```python
from build123d import *

# Parameters (mm, degrees)
F0_W     = 25.4
F0_H     = 25.4
F1_DEPTH = 25.4
F3_DEPTH = 25.4
F4_W     = 25.4
F4_H     = 12.7
F5_DEPTH = 25.4
F6_W     = 12.7
F6_H     = 12.7
F7_DEPTH = 25.4


with BuildPart() as f1:
    # F0 (on Front) → F1 (new body)
    with BuildSketch(Plane.XZ):
        with Locations((12.7, 12.7)):
            Rectangle(F0_W, F0_H)
    extrude(amount=F1_DEPTH)

    # F2 (on face) → F3 (cut)
    with BuildSketch(Plane.XZ.offset(25.4)):
        Polygon((5.187699, 9.677647), (0.70863, 9.677647), (0.70863, 7.712204), (1.221623, 7.712204), (1.221623, 4.225912), (0.734957, 4.225912), (0.734957, 2.289937), (3.984629, 2.289937), (3.984629, 4.225912), (3.45915, 4.225912), (3.45915, 4.571622), (5.187699, 4.571622), (6.487568, 5.940633), (6.487568, 8.277631), align=None)
        Polygon((1.373146, 8.298191), (1.373146, 9.056263), (4.895022, 9.024677), (5.842611, 8.09288), (5.842611, 6.181907), (4.942401, 5.234317), (2.826117, 5.234317), (2.826117, 3.623415), (3.284119, 3.623415), (3.284119, 2.928515), (1.373146, 2.928515), (1.373146, 3.623415), (1.89432, 3.623415), (1.89432, 8.298191), align=None, mode=Mode.SUBTRACT)
        Polygon((10.355519, 9.670121), (7.154135, 9.670121), (7.164647, 7.688757), (7.654916, 7.688757), (7.654916, 4.259461), (7.164647, 4.259461), (7.164647, 2.317117), (10.355519, 2.317117), (10.355519, 4.259461), (9.8595, 4.259461), (9.8595, 7.691912), (10.355519, 7.691912), align=None)
        Polygon((7.806116, 8.34365), (7.802438, 9.036948), (9.705184, 9.037424), (9.708923, 8.332776), (9.163893, 8.329884), (9.18893, 3.610964), (9.708865, 3.624296), (9.722495, 2.901242), (7.792784, 2.891004), (7.788839, 3.634657), (8.348879, 3.637628), (8.348879, 8.34653), align=None, mode=Mode.SUBTRACT)
        Polygon((13.681499, 9.670121), (11.003493, 9.670121), (11.003493, 7.688757), (11.510781, 7.688757), (11.510781, 4.259461), (11.003493, 4.259461), (11.003493, 2.317117), (13.988231, 2.317117), (13.988231, 4.166804), (13.351173, 4.166804), (13.351173, 5.936412), (15.344931, 2.317117), (17.279701, 2.317117), (17.279701, 7.688757), (17.810585, 7.688757), (17.810585, 9.670121), (14.908427, 9.670121), (14.908427, 7.800398), (15.403918, 7.800398), (15.403918, 6.420104), align=None)
        Polygon((11.66257, 8.332776), (11.658834, 9.036948), (13.255958, 9.006472), (15.985473, 4.235322), (15.985473, 8.338282), (15.528347, 8.332776), (15.520232, 9.006472), (17.214789, 9.026884), (17.218454, 8.336145), (16.583439, 8.332776), (16.611911, 2.966279), (15.742617, 2.961667), (12.90889, 8.117346), (12.932612, 3.646248), (13.373935, 3.648589), (13.377531, 2.970786), (11.682376, 2.961792), (11.679067, 3.58549), (12.16921, 3.588091), (12.144037, 8.332776), align=None, mode=Mode.SUBTRACT)
        Polygon((21.357853, 9.670121), (18.333804, 9.670121), (18.319575, 7.688901), (18.870167, 7.686202), (18.852962, 4.176179), (18.319575, 4.176179), (18.319575, 2.266313), (21.31342, 2.266313), (21.31342, 4.176179), (21.00371, 4.176179), (21.00371, 4.399857), (21.709157, 5.139715), (22.139307, 4.176179), (21.65754, 4.176179), (21.65754, 2.283519), (24.823442, 2.283519), (24.823442, 4.227797), (24.169615, 4.227797), (23.051225, 6.671048), (24.049172, 7.703408), (24.823442, 7.703408), (24.823442, 9.647685), (21.65754, 9.647685), (21.65754, 7.858261), (21.798439, 7.858261), (21.070654, 7.032285), (21.070654, 7.843203), (21.357853, 7.843203), align=None)
        Polygon((19.004352, 8.332776), (19.000616, 9.036948), (20.667763, 9.036053), (20.667763, 8.306677), (20.414714, 8.306677), (20.414714, 5.552904), (22.945207, 8.336446), (22.349797, 8.336446), (22.349797, 9.036053), (24.180682, 9.036053), (24.180682, 8.312229), (23.73184, 8.312229), (22.349797, 6.743724), (23.704356, 3.588185), (24.180682, 3.588185), (24.180682, 2.962871), (22.349797, 2.962871), (22.349797, 3.588185), (22.945207, 3.588185), (21.754388, 6.207855), (20.414714, 4.644904), (20.414714, 3.588185), (20.679095, 3.588185), (20.682522, 2.942261), (19.004326, 2.933357), (19.000867, 3.585446), (19.517002, 3.588185), (19.491829, 8.332776), align=None, mode=Mode.SUBTRACT)
        Polygon((4.895022, 9.024677), (1.373146, 9.056263), (1.373146, 8.298191), (1.89432, 8.298191), (1.89432, 3.623415), (1.373146, 3.623415), (1.373146, 2.928515), (3.284119, 2.928515), (3.284119, 3.623415), (2.826117, 3.623415), (2.826117, 5.234317), (4.942401, 5.234317), (5.842611, 6.181907), (5.842611, 8.09288), align=None)
        Polygon((9.705184, 9.037424), (7.802438, 9.036948), (7.806116, 8.34365), (8.348879, 8.34653), (8.348879, 3.637628), (7.788839, 3.634657), (7.792784, 2.891004), (9.722495, 2.901242), (9.708865, 3.624296), (9.18893, 3.610964), (9.163893, 8.329884), (9.708923, 8.332776), align=None)
        Polygon((13.255958, 9.006472), (11.658834, 9.036948), (11.66257, 8.332776), (12.144037, 8.332776), (12.16921, 3.588091), (11.679067, 3.58549), (11.682376, 2.961792), (13.377531, 2.970786), (13.373935, 3.648589), (12.932612, 3.646248), (12.90889, 8.117346), (15.742617, 2.961667), (16.611911, 2.966279), (16.583439, 8.332776), (17.218454, 8.336145), (17.214789, 9.026884), (15.520232, 9.006472), (15.528347, 8.332776), (15.985473, 8.338282), (15.985473, 4.235322), align=None)
        Polygon((20.667763, 9.036053), (19.000616, 9.036948), (19.004352, 8.332776), (19.491829, 8.332776), (19.517002, 3.588185), (19.000867, 3.585446), (19.004326, 2.933357), (20.682522, 2.942261), (20.679095, 3.588185), (20.414714, 3.588185), (20.414714, 4.644904), (21.754388, 6.207855), (22.945207, 3.588185), (22.349797, 3.588185), (22.349797, 2.962871), (24.180682, 2.962871), (24.180682, 3.588185), (23.704356, 3.588185), (22.349797, 6.743724), (23.73184, 8.312229), (24.180682, 8.312229), (24.180682, 9.036053), (22.349797, 9.036053), (22.349797, 8.336446), (22.945207, 8.336446), (20.414714, 5.552904), (20.414714, 8.306677), (20.667763, 8.306677), align=None)
    extrude(amount=-F3_DEPTH, mode=Mode.SUBTRACT)

    # F4 (on face) → F5 (cut)
    with BuildSketch(Plane.XZ.offset(25.4)):
        with Locations((12.7, 19.05)):
            Rectangle(F4_W, F4_H)
    extrude(amount=-F5_DEPTH, mode=Mode.SUBTRACT)

    # F6 (on face) → F7 (cut)
    with BuildSketch(Plane(origin=(0, 0, 0), x_dir=(0, -1, 0), z_dir=(-1, 0, 0))):
        with Locations((19.05, 6.35)):
            Rectangle(F6_W, F6_H)
    extrude(amount=-F7_DEPTH, mode=Mode.SUBTRACT)


solid = f1.part
```
Verification items for the finished model (mm, model axes). Give positions to 0.01 mm unless a question says otherwise; leave off trailing zeros. Order: outer loops, then holes, each group sorted by start corner. A loop starts at its lowest first (then second) coordinate and runs counter-clockwise, first axis right, second up. Notation, with made-up numbers: M 25.5,39.5 L 62.5,39.5 A25 cw 62.5,59.5 Z; hole C -16,-36 d4. An arc over 180 degrees is marked long. Return JSON: item names as keys, results as strings. Group by question number.
1) Go/stop test with a flat-tipped pin: pin 1 Ø4 at (y, z) = (-10.5, 2) entering from -X. Record where the tip stops, or that it passes through.
2) Section check A-A on x = 19.75. Record the cut outline in (y, z), and give its area (3 significant figures).
3) Section check C-C on x = 16.5. Record the cut outline in (y, z), and give its area (3 significant figures).
4) Scan lines: line 1 (Z direction, x = 10, y = -12); line 2 (Z direction, x = 17.75, y = -5.5); line 3 (Z direction, x = 7.75, y = -7.5). Record each from-to range of solid material in increasing order.
5) Section check D-D on y = -10.5. Give the number of separate pieces and of enclosed holes in the cut face, and give its area (3 significant figures).
6) Mould release check, pull along X, two halves, no side actions. Record for faces 1 (the face through (13, 0, 2)), 2 (the face through (24.823, -6, 9)): pulls with the +X half, pulls with the -X half, needs draft (parallel to the pull), parting line crosses it, or undercut.
7) Section check B-B on z = 5.5. Record the cut outline in (x, y).
Answer block:
{
 "1": {"pin 1": "stops at x = 0"},
 "2": {"outline": "M -12.7,0 L 0,0 L 0,2.27 L -12.7,2.27 Z; M -12.7,9.67 L 0,9.67 L 0,12.7 L -12.7,12.7 Z", "area": "67.3 mm^2"},
 "3": {"outline": "M -12.7,0 L 0,0 L 0,2.32 L -12.7,2.32 Z; M -12.7,9.67 L 0,9.67 L 0,12.7 L -12.7,12.7 Z", "area": "67.9 mm^2"},
 "4": {"line 1": "z = 0 to 2.32, 4.26 to 7.69, 9.67 to 12.7", "line 2": "z = 0 to 7.69, 9.67 to 12.7", "line 3": "z = 0 to 2.32, 9.67 to 12.7"},
 "5": {"separate pieces": "1", "enclosed holes": "4", "area": "188 mm^2"},
 "6": {"face 1": "needs draft", "face 2": "undercut"},
 "7": {"outline": "M 0,-12.7 L 1.22,-12.7 L 1.22,0 L 0,0 Z; M 6.07,-12.7 L 7.65,-12.7 L 7.65,0 L 6.07,0 Z; M 9.86,-12.7 L 11.51,-12.7 L 11.51,0 L 9.86,0 Z; M 13.35,-12.7 L 13.59,-12.7 L 13.59,0 L 13.35,0 Z; M 17.28,-12.7 L 18.86,-12.7 L 18.86,0 L 17.28,0 Z; M 23.59,-12.7 L 25.4,-12.7 L 25.4,0 L 23.59,0 Z"}
}
